Autodesk Fusion 360 part; units mm, degrees
sketch "Sketch1" plane through (0, 0, 0) normal (0, 0, 1) x (1, 0, 0)
  line L0 (0, 0) -> (40, 0)
  line L1 (40, 0) -> (40, 60)
  line L2 (40, 60) -> (0, 60)
  line L3 (0, 60) -> (0, 0)
  circle A0 centre (5, 5) radius 1.35
  circle A1 centre (20, 30) radius 7.25
  circle A2 centre (20, 30) radius 5.75
  circle A3 centre (35, 5) radius 1.35
  circle A4 centre (5, 30) radius 1.35
  circle A5 centre (35, 30) radius 1.35
  circle A6 centre (5, 55) radius 1.35
  circle A7 centre (35, 55) radius 1.35
  circle A8 centre (20, 6) radius 5
  line L4 (-10, 40) -> (50, 40)
  line L5 (50, 40) -> (50, 20)
  line L6 (50, 20) -> (-10, 20)
  line L7 (-10, 20) -> (-10, 40)
  circle A9 centre (-5, 30) radius 1.35
  circle A10 centre (45, 30) radius 1.35
  dimension "d1" = 2.7
  dimension "d2" = 60
  dimension "d3" = 40
  dimension "d4" = 5
  dimension "d5" = 5
  dimension "d6" = 14.5
  dimension "d7" = 20
  dimension "d8" = 30
  dimension "d9" = 11.5
  dimension "d12" = 30
  dimension "d13" = 50
  dimension "d20" = 6
  dimension "d21" = 20
  dimension "d22" = 10
  dimension "d23" = 60
  dimension "d24" = 20
  dimension "d25" = 30
  dimension "d26" = 10
  dimension "d29" = 50
  dimension "d30" = 0
  dimension "d31" = 2.7
  dimension "d32" = 5
  dimension "d33" = 10
extrude "Extrude1" add sketch "Sketch1" along normal blind 2 contours L0 L1 L3 L6 | L3 L4 L6 L7 | L1 L3 L4 L6 | L1 L4 L5 L6 | L1 L2 L3 L4
fillet "Fillet2" radius 2 4 edges at (40, 20, 1) (40, 40, 1) (0, 40, 1) (0, 20, 1)
sketch "Sketch2" plane through (0, 0, 2) normal (0, 0, 1) x (-1, 0, 0)
  circle A0 centre (-5, -5) radius 1.35
  circle A1 centre (-5, -30) radius 1.35
  circle A2 centre (-35, -5) radius 1.35
  circle A3 centre (-35, -30) radius 1.35
  circle A4 centre (-35, -55) radius 1.35
  circle A5 centre (-20, -6) radius 5
  circle A6 centre (-20, -30) radius 7.25
  circle A7 centre (-45, -30) radius 1.35
  circle A8 centre (5, -30) radius 1.35
  circle A9 centre (-5, -55) radius 1.35
  line L0 (0, -18) -> (0, 0)
  line L1 (0, 0) -> (-40, 0)
  line L2 (-40, 0) -> (-40, -18)
  arc A10 (-42, -20) -> (-40, -18) centre (-42, -18) ccw
  line L3 (-42, -20) -> (-50, -20)
  line L4 (-50, -20) -> (-50, -40)
  line L5 (-50, -40) -> (-42, -40)
  arc A11 (-40, -42) -> (-42, -40) centre (-42, -42) ccw
  line L6 (-40, -42) -> (-40, -60)
  line L7 (-40, -60) -> (0, -60)
  line L8 (0, -60) -> (0, -42)
  arc A12 (2, -40) -> (0, -42) centre (2, -42) ccw
  line L9 (2, -40) -> (10, -40)
  line L10 (10, -40) -> (10, -20)
  line L11 (10, -20) -> (2, -20)
  arc A13 (0, -18) -> (2, -20) centre (2, -18) ccw
  circle A14 centre (-5, -45) radius 2.5
  circle A15 centre (-35, -45) radius 2.5
  circle A16 centre (-5, -15) radius 2.5
  circle A17 centre (-35, -15) radius 2.5
  dimension "d38" = -30
  dimension "d39" = 30
  dimension "d40" = 5
  dimension "d41" = 15
  dimension "d42" = 5
extrude "Extrude3" cut sketch "Sketch2" against normal blind 2 contours A14 | A15 | A16 | A17
extrude "Extrude2" [suppressed]
fillet "Fillet1" [suppressed]
Geometry: final body of the model. Coordinates: model frame, mm. A direction names the side the tool comes from. Give positions to 0.01 mm unless a question says otherwise; leave off trailing zeros. Order: outer loops, then holes, each group sorted by start corner. A loop starts at its lowest first (then second) coordinate and runs counter-clockwise, first axis right, second up. Notation, with made-up numbers: M -17,-8 L 16,-8 A22 ccw 16,30 Z; hole C -17,65.25 d6. An arc over 180 degrees is marked long. Answer as CSV lines item,"result". Start each with the question number.
1) Cut plane B-B (x = 45). Output: boundary loops of the cut face in (y, z), then the cut area to 3 significant figures.
2) Cut plane A-A (x = 5). Output: boundary loops of the cut face in (y, z), then the cut area to 3 significant figures.
3) Line query: line 1 (Y direction, x = 5, z = 1.05); line 2 (X direction, y = 44, z = 1.3); line 3 (Y direction, x = 36, z = 1.25). Output: solid intervals per line, ascending. Write a range as from..to.
4) Set-up query: faces 1 (the flat face through (0, 9, 1)), 2 (the flat face through (0, 51, 1)), 3 (the flat face through (46, 20, 1)), 4 (the flat face through (46, 40, 1)), 5 (the cylindrical face through (32.69, 45.96, 1.01)). Return all of +Z, -Z, +X, -X, +Y, -Y with unobstructed straight access to the full face (end or side cutting, diameter ignored); none if empty.
5) Mould query, pull axis Y, two halves, no side actions, for faces 6 (the cylindrical face through (18.92, 10.88, 0.99)), 7 (the flat face through (20, 0, 1)), 8 (the flat face through (40, 9, 1)). Classes: +Y half, -Y half, draft (parallel to the pull), parting line (faces both ways), or undercut.
6) Cut plane C-C (z = 0.55). State how many separate pieces and enclosed holes the cut face has, then the cut area to 3 significant figures.
7) First-contact query: P1, Ø1.6, axis at x = -5, y = 30, coming from the +Z side; P2, Ø1, axis at y = 5.5, z = 1.5, coming from the +X side; P3, Ø3, axis at x = 11, y = 49, coming from the -Z side; P4, Ø1, axis at x = 46.5, z = 0.5, coming from the +Y side. Flat tips, straight axial feed; report the tip coordinate or a pass-through.
8) Cut plane D-D (y = 35). Output: boundary loops of the cut face in (x, z), then the cut area to 3 significant figures.
Findings below:
1,outline,"M 20,0 L 28.65,0 L 28.65,2 L 20,2 Z; M 31.35,0 L 40,0 L 40,2 L 31.35,2 Z"
1,area,"34.6 mm²"
2,outline,"M 0,0 L 3.65,0 L 3.65,2 L 0,2 Z; M 6.35,0 L 12.5,0 L 12.5,2 L 6.35,2 Z; M 17.5,0 L 28.65,0 L 28.65,2 L 17.5,2 Z; M 31.35,0 L 42.5,0 L 42.5,2 L 31.35,2 Z; M 47.5,0 L 53.65,0 L 53.65,2 L 47.5,2 Z; M 56.35,0 L 60,0 L 60,2 L 56.35,2 Z"
2,area,"83.8 mm²"
3,line 1,"y = 0..3.65, 6.35..12.5, 17.5..28.65, 31.35..42.5, 47.5..53.65, 56.35..60"
3,line 2,"x = 0..2.71, 7.29..32.71, 37.29..40"
3,line 3,"y = 0..4.09, 5.91..12.71, 17.29..29.09, 30.91..42.71, 47.29..54.09, 55.91..60"
4,face 1,"+Z, -Z, -X, -Y"
4,face 2,"+Z, -Z, -X, +Y"
4,face 3,"+Z, -Z, +X, -Y"
4,face 4,"+Z, -Z, +X, +Y"
4,face 5,"+Z, -Z"
5,face 6,"undercut"
5,face 7,"-Y half"
5,face 8,"draft"
6,separate pieces,"1"
6,enclosed holes,"14"
6,area,"2,440 mm²"
7,P1,"passes through"
7,P2,"stops at x = 40"
7,P3,"stops at z = 0"
7,P4,"stops at y = 40"
8,outline,"M -10,0 L 14.75,0 L 14.75,2 L -10,2 Z; M 25.25,0 L 50,0 L 50,2 L 25.25,2 Z"
8,area,"99.0 mm²"
